from build123d import *

# Parameters (mm, degrees)
IZIM1_R                     = 10
IZIM1_R_2                   = 1.5
Y_KSEKLIK_EKSTR_ZYON1_DEPTH = 2
IZIM2_R                     = 2.5
IZIM2_R_2                   = 1.724737241
Y_KSEKLIK_EKSTR_ZYON2_DEPTH = 2


with BuildPart() as part:
    # Çizim1 → Yükseklik-Ekstrüzyon1 (new body)
    with BuildSketch(Plane(origin=(0, 0, 0), x_dir=(1, 0, 0), z_dir=(0, 1, 0))):
        with Locations(Location((-0.153619206, 0.084194337, 0), (0, 0, 270))):
            Circle(IZIM1_R)
        with Locations(Location((-0.153619206, 0.084194337, 0), (0, 0, 270))):
            Circle(IZIM1_R_2, mode=Mode.SUBTRACT)
        with Locations(Location((-0.153619206, 5.084194337, 0), (0, 0, 270))):
            Circle(IZIM1_R_2, mode=Mode.SUBTRACT)
        with Locations(Location((-5.153619206, 0.084194337, 0), (0, 0, 270))):
            Circle(IZIM1_R_2, mode=Mode.SUBTRACT)
        with Locations(Location((4.846380794, 0.084194337, 0), (0, 0, 270))):
            Circle(IZIM1_R_2, mode=Mode.SUBTRACT)
        with Locations(Location((-0.153619206, -4.915805663, 0), (0, 0, 270))):
            Circle(IZIM1_R_2, mode=Mode.SUBTRACT)
    extrude(amount=Y_KSEKLIK_EKSTR_ZYON1_DEPTH)

    # Çizim2 → Yükseklik-Ekstrüzyon2 (add)
    with BuildSketch(Plane.XZ):
        with Locations(Location((-0.153619206, -0.084194337, 0), (0, 0, 90))):
            Circle(IZIM2_R)
        with Locations(Location((-0.153619206, -0.084194337, 0), (0, 0, 270))):
            Circle(IZIM2_R_2, mode=Mode.SUBTRACT)
    extrude(amount=Y_KSEKLIK_EKSTR_ZYON2_DEPTH)


solid = part.part
The model under review builds one solid part; all positions refer to its coordinate system, in mm. A direction names the side the tool comes from. Round coordinates to 2 decimals unless told otherwise and drop trailing zeros. Loops run counter-clockwise (first coordinate to the right, second up) from the corner with the lowest first, then second, coordinate; pieces in that order, holes last. Notation, with made-up numbers: (-8.5, -6) -> (28.5, -6) arc R11 ccw to (28.5, 0) -> close; hole circle Ø11 at (71, 23.25). An arc over 180 degrees is marked (long way). One line per question, with ' | ' between items. Start each with the question number.
Item 1: Draft analysis for pull direction Z (two halves, no side actions). For faces 3 (the face through (3.382, 0.986, -0.409)), 4 (the face through (-1, -2, 2)), 5 (the face through (-0.9, -1, 2.3)), state which applies: +Z half, -Z half, draft (parallel to the pull), parting line (faces both ways), or undercut.
Item 2: Add section B-B, the plane y = -0.95. Write out the cut boundary in (x, z), then the cut area to 3 significant figures.
Item 3: Add section C-C, the plane x = -6.25. Write out the cut boundary in (y, z), then the cut area to 3 significant figures.
Item 4: Add section A-A, the plane x = 5.75. Write out the cut boundary in (y, z).
Item 5: Machinability: for faces 1 (the face through (-2, 0, 2)), 2 (the face through (-0.088, 0.986, -6.583)), which of the approach directions +Z, -Z, +X, -X, +Y, -Y give a long, thin tool a straight path to every point of the face, cutting with its end or side? Answer none if there is none.
Item 6: Wall thickness on line 1 along X through (y, z) = (1.6, 1); line 2 along X through (y, z) = (1.35, 1.25); line 3 along Y through (x, z) = (5.75, 5): over which ranges is each line inside the solid? List them lowest first. Write a range as [from, to].
Item 7: Add section D-D, the plane y = 1.05. Write out the cut boundary in (x, z), then the cut area to 3 significant figures.
Item 8: For pin 1 (3.5 mm diameter, centred on x = -0.15, z = 4.92, fed in from -Y); pin 2 (1.5 mm diameter, centred on y = 0.5, z = -3, fed in from +X); pin 3 (1.5 mm diameter, centred on y = 0.5, z = 1.5, fed in from +X), all flat-tipped, find the tip position at first contact; note any pin that passes through.
Return value:
1) face 3: undercut | face 4: draft | face 5: parting line
2) outline: circle Ø5 at (-0.15, -0.08); hole circle Ø3.45 at (-0.15, -0.08) | area: 10.3 mm2
3) outline: (0, -8.01) -> (2, -8.01) -> (2, -1.11) -> (0, -1.11) -> close; (0, 0.94) -> (2, 0.94) -> (2, 7.84) -> (0, 7.84) -> close | area: 27.6 mm2
4) outline: (0, -8.16) -> (2, -8.16) -> (2, -1.28) -> (0, -1.28) -> close; (0, 1.11) -> (2, 1.11) -> (2, 7.99) -> (0, 7.99) -> close
5) face 1: -Y | face 2: +Y, -Y
6) line 1: x = [-10.09, -6.19], [-4.12, -1.19], [0.88, 3.81], [5.88, 9.79] | line 2: x = [-10.06, -5.84], [-4.47, -0.84], [0.53, 4.16], [5.53, 9.76] | line 3: y = [0, 2]
7) outline: circle Ø20 at (-0.15, -0.08); hole circle Ø3 at (-5.15, -0.08); hole circle Ø3 at (-0.15, -5.08); hole circle Ø3 at (-0.15, -0.08); hole circle Ø3 at (-0.15, 4.92); hole circle Ø3 at (4.85, -0.08) | area: 279 mm2
8) pin 1: stops at y = 0 | pin 2: stops at x = 9.61 | pin 3: stops at x = 9.81
